Geometry check sheet. Reference: the model listing, model coordinates, mm. Face numbers are marked on the shaded views. Give positions to 0.01 mm unless a question says otherwise; leave off trailing zeros. Order: outer loops, then holes, each group sorted by start corner. A loop starts at its lowest first (then second) coordinate and runs counter-clockwise, first axis right, second up.
```python
from build123d import *

# Parameters (mm, degrees)
SKETCH1_W           = 30
SKETCH1_H           = 45
BOSS_EXTRUDE1_DEPTH = 5
SKETCH2_R           = 4
CUT_EXTRUDE1_DEPTH  = 5
SKETCH3_R           = 1.55
CUT_EXTRUDE2_DEPTH  = 5
SKETCH4_R           = 0.8
CUT_EXTRUDE3_DEPTH  = 5
SKETCH5_R           = 2.5
BOSS_EXTRUDE2_DEPTH = 10
FILLET1_R           = 2


with BuildPart() as part:
    # Sketch1 → Boss-Extrude1 (new body)
    with BuildSketch(Plane(origin=(0, 0, 0), x_dir=(1, 0, 0), z_dir=(0, 1, 0))):
        with Locations((7.687417977, 3.694491888)):
            Rectangle(SKETCH1_W, SKETCH1_H)
    extrude(amount=BOSS_EXTRUDE1_DEPTH)

    # Sketch2 → Cut-Extrude1 (cut)
    with BuildSketch(Plane(origin=(0, 5, 0), x_dir=(-1, 0, 0), z_dir=(0, 1, 0))):
        with Locations(Location((-7.687417977, -11.194491888, 0), (0, 0, 90))):
            Circle(SKETCH2_R)
    extrude(amount=-CUT_EXTRUDE1_DEPTH, mode=Mode.SUBTRACT)

    # Sketch3 → Cut-Extrude2 (cut)
    with BuildSketch(Plane(origin=(0, 5, 0), x_dir=(1, 0, 0), z_dir=(0, 1, 0))):
        with Locations(Location((2.030563727, 16.851346138, 0), (0, 0, 270))):
            Circle(SKETCH3_R)
        with Locations(Location((14.404932398, 17.912006309, 0), (0, 0, 270))):
            Circle(SKETCH3_R)
        with Locations(Location((13.344272226, 5.537637639, 0), (0, 0, 270))):
            Circle(SKETCH3_R)
        with Locations(Location((0.969903556, 4.476977467, 0), (0, 0, 270))):
            Circle(SKETCH3_R)
    extrude(amount=-CUT_EXTRUDE2_DEPTH, mode=Mode.SUBTRACT)

    # Sketch4 → Cut-Extrude3 (cut)
    with BuildSketch(Plane.XY.offset(18.805508112)):
        with Locations((-2.812582023, 2.5)):
            Circle(SKETCH4_R)
        with Locations((18.187417977, 2.5)):
            Circle(SKETCH4_R)
    extrude(amount=-CUT_EXTRUDE3_DEPTH, mode=Mode.SUBTRACT)

    # Sketch5 → Boss-Extrude2 (add)
    with BuildSketch(Plane(origin=(0, 0, -26.194491888), x_dir=(-1, 0, 0), z_dir=(0, 0, -1))):
        with Locations(Location((-7.687417977, 2.5, 0), (0, 0, 270))):
            Circle(SKETCH5_R)
    extrude(amount=BOSS_EXTRUDE2_DEPTH)

    # Fillet1
    fillet1_edges = [part.edges().sort_by_distance(p)[0] for p in [
        (-7.312582023, 5, -3.694491888),
        (22.687417977, 5, -3.694491888),
        (-7.312582023, 0, -3.694491888),
        (22.687417977, 0, -3.694491888),
    ]]
    fillet(fillet1_edges, radius=FILLET1_R)


solid = part.part
```
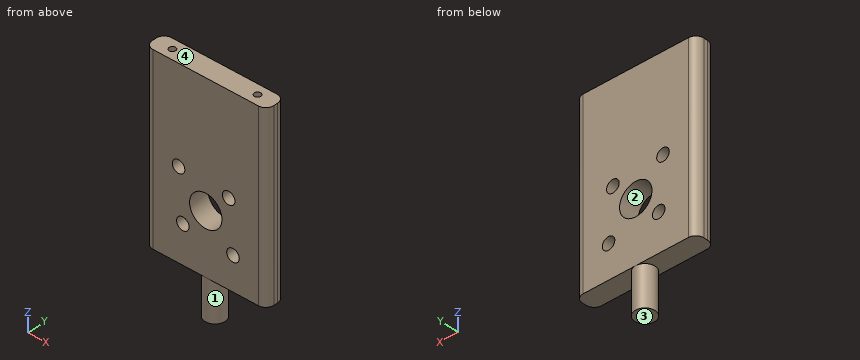
Q1. Cross-section at A-A, the plane z = -23. Record the boundary of the cut face in (x, y).
Q2. Release check for a two-part mould opening along Z. For the marked faces 1, 2, 3 and 4 record: pulls with the +Z half, pulls with the -Z half, needs draft (parallel to the pull), parting line crosses it, or undercut.
Q3. Cross-section at B-B, the plane x = 9.5. Record the boundary of the cut face in (y, z).
Q4. Cross-section at D-D, the plane z = -8. Record the boundary of the cut face in (x, y).
Q5. Thickness scan on L1, parallel to Z at x = 14.75, y = 1.9; L2, parallel to Z at x = -2, y = 1.2; L3, parallel to Z at x = 14.25, y = 2.55. Record the ranges inside material, lowest first.
Q6. Cross-section at C-C, the plane y = 4.45. Record the boundary of the cut face in (x, z), and give its area (3 significant figures).
Q7. Gauge pin test, flat ends, axial feed: P1, Ø4, axis at x = 4.5, z = -29, coming from the +Y side; P2, Ø1.4, axis at x = 18.19, y = 2.5, coming from the +Z side; P3, Ø1, axis at y = 3.5, z = -28, coming from the -X side. Record the tip position at first contact, or that the pin passes through.
Answers follow:
1. outline: (-7.31, 2) arc R2 ccw to (-5.31, 0) - (20.69, 0) arc R2 ccw to (22.69, 2) - (22.69, 3) arc R2 ccw to (20.69, 5) - (-5.31, 5) arc R2 ccw to (-7.31, 3) - close
2. face 1: needs draft
2. face 2: undercut
2. face 3: pulls with the -Z half
2. face 4: pulls with the +Z half
3. outline: (0, -26.19) - (0.78, -26.19) - (0.78, -36.19) - (4.22, -36.19) - (4.22, -26.19) - (5, -26.19) - (5, -14.76) - (0, -14.76) - close; (0, -7.63) - (5, -7.63) - (5, 18.81) - (0, 18.81) - close
4. outline: (-7.31, 2) arc R2 ccw to (-5.31, 0) - (5.28, 0) - (5.28, 5) - (-5.31, 5) arc R2 ccw to (-7.31, 3) - close; (10.09, 0) - (20.69, 0) arc R2 ccw to (22.69, 2) - (22.69, 3) arc R2 ccw to (20.69, 5) - (10.09, 5) - close
5. L1: z = -26.19 to -19.42, -16.4 to -6.19, -4.88 to 18.81
5. L2: z = -26.19 to 18.81
5. L3: z = -26.19 to -19.45, -16.37 to -6.8, -4.28 to 18.81
6. outline: (-6.69, -26.19) - (6.12, -26.19) - (6.12, -36.19) - (9.25, -36.19) - (9.25, -26.19) - (22.06, -26.19) - (22.06, 18.81) - (-6.69, 18.81) - close; hole circle Ø3.1 at (0.97, -4.48); hole circle Ø3.1 at (2.03, -16.85); hole circle Ø8 at (7.69, -11.19); hole circle Ø3.1 at (13.34, -5.54); hole circle Ø3.1 at (14.4, -17.91)
6. area: 1,240 mm2
7. P1: stops at y = 4.7
7. P2: stops at z = 13.81
7. P3: stops at x = 5.24
